Part model, mm, in its own coordinate system. A direction names the side the tool comes from. Coordinates: 2 decimals unless noted, no trailing zeros. Answer in a Markdown table with one row per item. Add a question column.
from build123d import *

# Parameters (mm, degrees)
BODY_SKETCH_R                           = 53
BODY_SKETCH_R_2                         = 43.5
BODY_DEPTH                              = 25
SIDE_CUTOUTS_DEPTH                      = 80.012657213892
DRIVING_CUTOUT_DEPTH                    = 80.012657213892
DRIVING_CUTOUT_FILLET_R                 = 0.25
MAIN_PATTERN_COUNT                      = 6
DRIVING_CUTOUT_FILLET_OF_MAIN_PATTERN_R = 0.25
OVERALL_CHAMFER_SIZE                    = 0.5


with BuildPart() as part:
    # body_sketch → body (new body)
    with BuildSketch(Plane(origin=(0, 0, 0), x_dir=(1, 0, 0), z_dir=(0, 1, 0))):
        with Locations(Location((0, 0, 0), (0, 0, 270))):
            Circle(BODY_SKETCH_R)
        with Locations(Location((0, 0, 0), (0, 0, 270))):
            Circle(BODY_SKETCH_R_2, mode=Mode.SUBTRACT)
    extrude(amount=BODY_DEPTH)

    # Sketch4 → spring_screw_hole (revolve, cut)
    with BuildSketch(Plane(origin=(48, 25, 0), x_dir=(0, 0, 1), z_dir=(1, 0, 0))):
        Polygon((0, 0), (-6.12e-15, 25), (1.6999999999999937, 25), (1.6999999999999953, 20), (3.249999999999998, 20), (3.2499999999999996, 0.02500000000000014), (3.2750000000000004, -3.47e-15), align=None)
    spring_screw_hole = revolve(axis=Axis((48, 31.34999999999999, 0), (0, -1, 0)), mode=Mode.SUBTRACT)

    # Sketch5 → side_cutouts (cut, through all)
    with BuildSketch(Plane(origin=(0, 25, 0), x_dir=(1, 0, 0), z_dir=(0, 1, 0))):
        with BuildLine():
            Line((50.50367150582007, 7.0978281489633614), (52.63160922139086, 6.238085504929012))
            ThreePointArc((52.63160922139086, 6.238085504929012), (45.89934640057521, 26.50000000000007), (31.718145128943295, 42.461267875315386))
            Line((31.718145128943295, 42.461267875315386), (31.398735241608467, 40.188548433942906))
            ThreePointArc((31.398735241608467, 40.188548433942906), (44.16729559300632, 25.50000000000007), (50.50367150582007, 7.0978281489633614))
        make_face()
    side_cutouts = extrude(amount=-SIDE_CUTOUTS_DEPTH, mode=Mode.SUBTRACT)

    # Sketch6 → driving_cutout (cut, through all)
    with BuildSketch(Plane(origin=(0, 25, 0), x_dir=(1, 0, 0), z_dir=(0, 1, 0))):
        Polygon((39.180373410532546, 18.898368697092206), (35.95665408703264, 24.48201435473557), (37.03918584176319, 25.107014354735572), (40.26290516526309, 19.52336869709221), align=None)
    driving_cutout = extrude(amount=-DRIVING_CUTOUT_DEPTH, mode=Mode.SUBTRACT)

    # driving_cutout_fillet
    driving_cutout_fillet_edges = [part.edges().sort_by_distance(p)[0] for p in [
        (40.26290516526309, 12.5, -19.52336869709221),
        (37.03918584176319, 12.5, -25.107014354735572),
    ]]
    fillet(driving_cutout_fillet_edges, radius=DRIVING_CUTOUT_FILLET_R)

    # main_pattern: spring_screw_hole, side_cutouts, driving_cutout ×6 about axis
    main_pattern_axis = Axis((-6.81e-15, 0, -3.023e-14), (0, 1, 0))
    add([spring_screw_hole.rotate(main_pattern_axis, i * 360 / MAIN_PATTERN_COUNT) for i in range(1, MAIN_PATTERN_COUNT)], mode=Mode.SUBTRACT)
    add([side_cutouts.rotate(main_pattern_axis, i * 360 / MAIN_PATTERN_COUNT) for i in range(1, MAIN_PATTERN_COUNT)], mode=Mode.SUBTRACT)
    add([driving_cutout.rotate(main_pattern_axis, i * 360 / MAIN_PATTERN_COUNT) for i in range(1, MAIN_PATTERN_COUNT)], mode=Mode.SUBTRACT)

    # driving_cutout_fillet of main_pattern
    driving_cutout_fillet_of_main_pattern_edges = [part.edges().sort_by_distance(p)[0] for p in [
        (3.223719323499823, 12.5, -44.63038305182766),
        (-3.223719323499948, 12.5, -44.63038305182764),
        (-37.03918584176327, 12.5, -25.10701435473548),
        (-40.26290516526315, 12.5, -19.523368697092106),
        (-40.262905165263106, 12.5, 19.523368697092145),
        (-37.03918584176321, 12.5, 25.107014354735508),
        (-3.2237193234998545, 12.5, 44.630383051827586),
        (3.223719323499913, 12.5, 44.63038305182758),
        (37.03918584176327, 12.5, 25.107014354735416),
        (40.26290516526314, 12.5, 19.523368697092028),
    ]]
    fillet(driving_cutout_fillet_of_main_pattern_edges, radius=DRIVING_CUTOUT_FILLET_OF_MAIN_PATTERN_R)

    # overall_chamfer
    overall_chamfer_edges = [part.edges().sort_by_distance(p)[0] for p in [
        (-26.50000000000005, 25, -45.89934640057521),
        (-53, 25, 4.441e-14),
        (-26.49999999999998, 25, 45.89934640057526),
        (26.50000000000005, 25, 45.89934640057522),
        (53, 25, -8.882e-14),
        (-26.500000000000234, 0, -45.89934640057511),
        (-53, 0, 3.4461e-13),
        (-26.499999999999897, 0, 45.899346400575304),
        (26.499999999999336, 0, 45.89934640057564),
        (53, 0, -7.6383e-13),
        (-4.866e-14, 0, -51),
        (-20.00920017832957, -3.55e-15, -47.992864981575195),
        (20.009200178329486, -3.55e-15, -47.99286498157525),
        (-4.828e-14, 25, -51.00000000000001),
        (20.009200178329486, 25, -47.992864981575245),
        (-20.00920017832958, 25, -47.992864981575195),
        (-44.16729559300637, 0, -25.499999999999982),
        (-51.56764036360546, 0, -6.6679568269460905),
        (-31.558440185275984, 0, -41.3249081546291),
        (-44.16729559300637, 25, -25.499999999999986),
        (-31.558440185275984, 25, -41.3249081546291),
        (-51.56764036360547, 25, -6.667956826946094),
        (-44.167295593006365, 0, 25.499999999999954),
        (-31.5584401852759, -3.55e-15, 41.32490815462907),
        (-51.56764036360548, 0, 6.667956826946121),
        (-44.16729559300633, 25, 25.49999999999999),
        (-51.56764036360548, 25, 6.66795682694612),
        (-31.5584401852759, 25, 41.32490815462907),
        (1.728e-14, 0, 50.99999999999995),
        (20.009200178329543, 0, 47.99286498157514),
        (-20.009200178329515, -3.55e-15, 47.99286498157518),
        (1.334e-14, 25, 50.99999999999994),
        (-20.009200178329515, 25, 47.99286498157518),
        (20.009200178329543, 25, 47.99286498157514),
        (44.167295593006365, 0, 25.499999999999908),
        (51.56764036360546, 0, 6.667956826946016),
        (31.55844018527599, 0, 41.324908154629036),
        (44.167295593006365, 25, 25.499999999999908),
        (31.558440185275984, 25, 41.324908154629036),
        (51.567640363605456, 25, 6.667956826946016),
        (-21.750000000000043, 25, -37.67210506462306),
        (-43.5, 25, 2.753e-14),
        (-21.74999999999997, 25, 37.672105064623096),
        (21.75000000000005, 25, 37.672105064623054),
        (43.5, 25, -7.994e-14),
        (26.499999999999932, 25, -45.89934640057529),
        (26.499999999999876, 0, -45.899346400575325),
        (44.167295593006315, 0, -25.500000000000057),
        (31.55844018527588, -3.55e-15, -41.32490815462914),
        (51.56764036360546, 0, -6.667956826946186),
        (44.167295593006315, 25, -25.500000000000057),
        (51.56764036360546, 25, -6.667956826946186),
        (31.55844018527588, 25, -41.32490815462914),
        (21.74999999999994, 25, -37.67210506462312),
    ]]
    chamfer(overall_chamfer_edges, length=OVERALL_CHAMFER_SIZE)


solid = part.part
(1) Wall check: line 1 (X direction, y = 2.9, z = 0); line 2 (X direction, y = 9.25, z = 0); line 3 (Z direction, x = -31, y = 2.5). Give the ranges that are in metal, low to high.
(2) Pull direction X, two halves, no side cores. Call faces 4 (the flat face through (-31.56, 12.67, 41.34)), 5 (the flat face through (43, 0, -8)), 6 (the cylindrical face through (43.5, 12.1, 0.3)), 7 (the conical face through (26.27, 24.809, -45.675)): pulls with the +X half, pulls with the -X half, needs draft (parallel to the pull), parting line crosses it, or undercut.
(3) Slice it at A-A (x = 24). State how many separate pieces and enclosed holes the cut face has, and give its area (3 significant figures).
(4) 3-axis set-ups, long thin cutter, end or side, ignore diameter. For faces 1 (the cylindrical face through (-21.987, 12.078, 37.535)), 2 (the conical face through (-21.58, 24.64, -37.93)), 3 (the cylindrical face through (-26.576, 12.332, 45.856)): which of +Z, -Z, +X, -X, +Y, -Y reach the whole face in a straight line?
(5) Drop flat-ended pins along their axis: P1, Ø2, axis at x = 48, z = 0, coming from the +Y side; P2, Ø1.9, axis at x = -25, z = -43, coming from the +Y side; P3, Ø2, axis at y = 9.5, z = 11, coming from the -X side; P4, Ø2, axis at y = 22, z = 2, coming from the -X side. Give the stop position or say it passes through.
Computed:
| question | item | result |
|---|---|---|
| 1 | line 1 | x = -53 to -49.7, -46.3 to -43.5, 43.5 to 46.3, 49.7 to 53 |
| 1 | line 2 | x = -53 to -51.25, -44.75 to -43.5, 43.5 to 44.75, 51.25 to 53 |
| 1 | line 3 | z = -42.99 to -30.52, 30.52 to 42.99 |
| 2 | face 4 | pulls with the -X half |
| 2 | face 5 | needs draft |
| 2 | face 6 | undercut |
| 2 | face 7 | pulls with the +X half |
| 3 | separate pieces | 4 |
| 3 | enclosed holes | 0 |
| 3 | area | 254 mm^2 |
| 4 | face 1 | +Y, -Y |
| 4 | face 2 | +Y |
| 4 | face 3 | +Z, -X, +Y, -Y |
| 5 | P1 | passes through |
| 5 | P2 | stops at y = 5 |
| 5 | P3 | stops at x = -50.01 |
| 5 | P4 | stops at x = -52.99 |
